from build123d import *

# Parameters (mm, degrees)
SKETCH1_R                = 12.5
BOSS_EXTRUDE1_DEPTH      = 20
SKETCH2_R                = 6
CUT_EXTRUDE2_DEPTH       = 56
BOSS_EXTRUDE2_DEPTH      = 5
BOSS_EXTRUDE2_DEPTH_BACK = 5


with BuildPart() as part:
    # Sketch1 → Boss-Extrude1 (new, symmetric)
    with BuildSketch(Plane.XY):
        with BuildLine():
            Line((-68.381118609, -39.565472128), (-68.381118609, 3.575463228))
            ThreePointArc((-68.381118609, 3.575463228), (-65.381118609, 67.434527872), (-62.381118609, 3.575463228))
            Line((-62.381118609, 3.575463228), (-62.381118609, -39.565472128))
            Line((-62.381118609, -39.565472128), (-37.381118609, -39.565472128))
            Line((-37.381118609, -39.565472128), (-37.381118609, -5.990102483))
            ThreePointArc((-37.381118609, -5.990102483), (-22.451762335, 9.801143977), (-15.631746753, 30.434527872))
            Line((-15.631746753, 30.434527872), (10.123983964, 30.434527872))
            ThreePointArc((10.123983964, 30.434527872), (59.618881391, 35.434527872), (10.123983964, 40.434527872))
            Line((10.123983964, 40.434527872), (-15.631746753, 40.434527872))
            ThreePointArc((-15.631746753, 40.434527872), (-91.014502504, 78.363884146), (-93.381118609, -5.990102483))
            Line((-93.381118609, -5.990102483), (-93.381118609, -39.565472128))
            Line((-93.381118609, -39.565472128), (-68.381118609, -39.565472128))
        make_face()
        with Locations((34.618881391, 35.434527872)):
            Circle(SKETCH1_R, mode=Mode.SUBTRACT)
    extrude(amount=BOSS_EXTRUDE1_DEPTH, both=True)

    # Sketch2 → Cut-Extrude2 (cut)
    with BuildSketch(Plane(origin=(-37.381118609, 0, 0), x_dir=(0, 0, -1), z_dir=(1, 0, 0))):
        with Locations((0, -22.777787305)):
            Circle(SKETCH2_R)
    extrude(amount=-CUT_EXTRUDE2_DEPTH, mode=Mode.SUBTRACT)

    # Sketch7 → Boss-Extrude2 (add, two sides: drawn at the far end of the back side and taken through both)
    with BuildSketch(Plane.XY.offset(-BOSS_EXTRUDE2_DEPTH_BACK)):
        with BuildLine():
            ThreePointArc((10.123983964, 40.434527872), (18.807493091, 54.799444603), (34.618881391, 60.434527872))
            Line((34.618881391, 60.434527872), (-22.079848419, 60.434527872))
            ThreePointArc((-22.079848419, 60.434527872), (-17.793247294, 50.777099487), (-15.631746753, 40.434527872))
            Line((-15.631746753, 40.434527872), (10.123983964, 40.434527872))
        make_face()
        with BuildLine():
            Line((-22.079848419, 10.434527872), (34.618881391, 10.434527872))
            ThreePointArc((34.618881391, 10.434527872), (18.807493091, 16.069611141), (10.123983964, 30.434527872))
            Line((10.123983964, 30.434527872), (-15.631746753, 30.434527872))
            ThreePointArc((-15.631746753, 30.434527872), (-17.793247294, 20.091956256), (-22.079848419, 10.434527872))
        make_face()
    extrude(amount=BOSS_EXTRUDE2_DEPTH + BOSS_EXTRUDE2_DEPTH_BACK)


solid = part.part
Work out the finished part from the listing and answer in its coordinate system (mm). A direction names the side the tool comes from. Coordinates: 2 decimals unless noted, no trailing zeros. Write each loop counter-clockwise with the first axis right and the second up, starting at its lowest first coordinate (ties: lowest second). Pieces come first, ordered by that corner, then holes. Notation, with made-up numbers: M 37.5,14 L 73.5,14 A22 cw 73.5,49 Z; hole C 50.5,12 d8. An arc over 180 degrees is marked long. Answer as CSV lines item,"result". Start each with the question number.
Item 1: Section D-D on x = 32.5 is taken. Write down the section's boundary in (y, z), and give its area (3 significant figures).
Item 2: Section B-B on z = 0 is taken. Write down the section's boundary in (x, y), and give its area (3 significant figures).
Item 3: Determine the mould class of faces 4 (the face through (25.406, 43.883, -0.28)), 5 (the face through (0, 53, 5)), 6 (the face through (-3, 30.435, 13)) for opening direction Y: released by +Y, released by -Y, zero draft, split by the parting line, or undercut.
Item 4: A tool of negligible diameter and unlimited length cuts with its end or side. For faces 1 (the face through (-3, 40.435, 13)), 2 (the face through (59.598, 34.406, 0.28)), 3 (the face through (-3, 30.435, -12)), from which of +Z, -Z, +X, -X, +Y, -Y can it reach the whole face along a straight path? Write none if from no direction.
Item 5: Section C-C on y = 15.5 is taken. Write down the section's boundary in (x, z), and give its area (3 significant figures).
Item 6: Consider L1, parallel to X at y = 35, z = 14; L2, parallel to X at y = -12, z = -10; L3, parallel to Y at x = -83, z = -5. Determine where each line is inside the solid, lowest interval first.
Item 7: Flat-ended cylindrical pins translate along their axes: P1, Ø4.5, axis at x = -3, z = -9, coming from the -Y side; P2, Ø12, axis at x = -11, z = -3, coming from the +Y side; P3, Ø20, axis at y = -8.5, z = 8, coming from the -X side; P4, Ø11, axis at y = -22.78, z = 0, coming from the +X side. Find the tip coordinate at first contact, or state that the pin passes through.
Item 8: Section A-A on x = -46 is taken. Write down the section's boundary in (y, z).
Checks:
1,outline,"M 10.43,-5 L 10.52,-5 L 10.52,-20 L 23.12,-20 L 23.12,20 L 10.52,20 L 10.52,5 L 10.43,5 Z; M 47.75,-20 L 60.34,-20 L 60.34,-5 L 60.43,-5 L 60.43,5 L 60.34,5 L 60.34,20 L 47.75,20 Z"
1,area,"1,010 mm²"
2,outline,"M -93.38,-39.57 L -68.38,-39.57 L -68.38,-28.78 L -93.38,-28.78 Z; M -93.38,-16.78 L -68.38,-16.78 L -68.38,3.58 A32 cw long -62.38,3.58 L -62.38,-16.78 L -37.38,-16.78 L -37.38,-5.99 A50 ccw -22.08,10.43 L 34.62,10.43 A25 ccw 34.62,60.43 L -22.08,60.43 A50 ccw long -93.38,-5.99 Z; M -62.38,-39.57 L -37.38,-39.57 L -37.38,-28.78 L -62.38,-28.78 Z; hole C 34.62,35.43 d25"
2,area,"8,430 mm²"
3,face 4,"undercut"
3,face 5,"zero draft"
3,face 6,"released by -Y"
4,face 1,"+Z, +Y"
4,face 2,"none"
4,face 3,"-Z, -Y"
5,outline,"M -111.24,-20 L -90.41,-20 L -90.41,20 L -111.24,20 Z; M -40.35,-20 L -19.53,-20 L -19.53,-5 L 19.53,-5 L 19.53,-20 L 49.71,-20 L 49.71,20 L 19.53,20 L 19.53,5 L -19.53,5 L -19.53,20 L -40.35,20 Z"
5,area,"3,260 mm²"
6,L1,"x = -115.38 to -97.38, -33.38 to 22.13, 47.11 to 59.62"
6,L2,"x = -93.38 to -68.38, -62.38 to -37.38"
6,L3,"y = -39.57 to -26.09, -19.46 to 8.72, 62.15 to 82.23"
7,P1,"stops at y = 30.43"
7,P2,"stops at y = 60.43"
7,P3,"stops at x = -102.1"
7,P4,"passes through"
8,outline,"M -39.57,-20 L 9.97,-20 L 9.97,20 L -39.57,20 Z; M 60.9,-20 L 81.53,-20 L 81.53,20 L 60.9,20 Z; hole C -22.78,0 d12"
